For this review, take the finished solid that the model builds, in its own axes (mm). Round coordinates to 2 decimals unless told otherwise and drop trailing zeros. Write each loop counter-clockwise with the first axis right and the second up, starting at its lowest first coordinate (ties: lowest second). Pieces come first, ordered by that corner, then holes. Notation, with made-up numbers: (56.5, 72) -> (64.5, 72) arc R17 cw to (64.5, 80) -> close; hole circle Ø7 at (34, 14.5). An arc over 180 degrees is marked (long way). Answer in a Markdown table with one row per item. Add a question column.
```python
from build123d import *

# Parameters (mm, degrees)
SKETCH1_R           = 1.5
BOSS_EXTRUDE1_DEPTH = 2
FILLET1_R           = 3


with BuildPart() as part:
    # Sketch1 → Boss-Extrude1 (new body)
    with BuildSketch(Plane.XY):
        with BuildLine():
            Line((-18, 29.5), (-18, -33.5))
            Line((-18, -33.5), (18, -33.5))
            Line((18, -33.5), (18, 29.5))
            ThreePointArc((18, 29.5), (17.746918084, 40.89430747), (16.988171513, 52.266140956))
            ThreePointArc((16.988171513, 52.266140956), (16.025040386, 54.213416236), (14, 55))
            Line((14, 55), (-14, 55))
            ThreePointArc((-14, 55), (-16.025040386, 54.213416236), (-16.988171513, 52.266140956))
            ThreePointArc((-16.988171513, 52.266140956), (-17.746918084, 40.89430747), (-18, 29.5))
        make_face()
        with Locations((-14, 29.5)):
            Circle(SKETCH1_R, mode=Mode.SUBTRACT)
        with Locations((14, 29.5)):
            Circle(SKETCH1_R, mode=Mode.SUBTRACT)
        with Locations((-14, -29.5)):
            Circle(SKETCH1_R, mode=Mode.SUBTRACT)
        with Locations((14, -29.5)):
            Circle(SKETCH1_R, mode=Mode.SUBTRACT)
        with Locations((15, 15)):
            Circle(SKETCH1_R, mode=Mode.SUBTRACT)
        with Locations((15, -15)):
            Circle(SKETCH1_R, mode=Mode.SUBTRACT)
        with Locations((-15, -15)):
            Circle(SKETCH1_R, mode=Mode.SUBTRACT)
        with Locations((-15, 15)):
            Circle(SKETCH1_R, mode=Mode.SUBTRACT)
        with Locations((-13, 52)):
            Circle(SKETCH1_R, mode=Mode.SUBTRACT)
        with Locations((13, 52)):
            Circle(SKETCH1_R, mode=Mode.SUBTRACT)
    extrude(amount=BOSS_EXTRUDE1_DEPTH)

    # Fillet1
    fillet1_edges = [part.edges().sort_by_distance(p)[0] for p in [
        (18, -33.5, 1),
        (-18, -33.5, 1),
    ]]
    fillet(fillet1_edges, radius=FILLET1_R)


solid = part.part
```
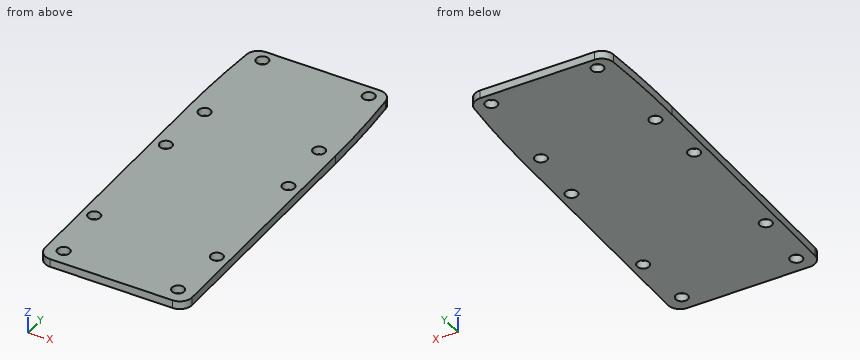
1. For L1, parallel to Y at x = -15, z = 0.7; L2, parallel to Y at x = 13, z = 1.55; L3, parallel to Y at x = 16, z = 1.55, list the stretches that pass through material, from the lowest coordinate up. Write a range as [from, to].
2. We need section A-A (z = 0.7). Count the separate pieces of the cut face and the enclosed holes in it, plus the area to 3 significant figures.
3. We need section B-B (y = 15). Write out the cut boundary in (x, z), plus the area to 3 significant figures.
Response:
| question | item | result |
|---|---|---|
| 1 | L1 | [-33.5, -30.62], [-28.38, -16.5], [-13.5, 13.5], [16.5, 28.38], [30.62, 54.83] |
| 1 | L2 | [-33.5, -30.62], [-28.38, 28.38], [30.62, 50.5], [53.5, 55] |
| 1 | L3 | [-33.33, -16.12], [-13.88, 13.88], [16.12, 54.24] |
| 2 | separate pieces | 1 |
| 2 | enclosed holes | 10 |
| 2 | area | 3,090 mm2 |
| 3 | outline | (-18, 0) -> (-16.5, 0) -> (-16.5, 2) -> (-18, 2) -> close; (-13.5, 0) -> (13.5, 0) -> (13.5, 2) -> (-13.5, 2) -> close; (16.5, 0) -> (18, 0) -> (18, 2) -> (16.5, 2) -> close |
| 3 | area | 60.0 mm2 |
